from build123d import *

# Parameters (mm, degrees)
SKETCH_1_W          = 141
SKETCH_1_H          = 80
EXTRUDE_1_DEPTH     = 3
SKETCH_2_R          = 1.5
CUT_EXTRUDE_1_DEPTH = 4
SKETCH_3_R          = 1.5
CUT_EXTRUDE_2_DEPTH = 4


with BuildPart() as part:
    # ｽｹｯﾁ1 → ﾎﾞｽ - 押し出し1 (new body)
    with BuildSketch(Plane(origin=(0, 0, 0), x_dir=(1, 0, 0), z_dir=(0, 1, 0))):
        with Locations((-70.5, 40)):
            Rectangle(SKETCH_1_W, SKETCH_1_H)
    extrude(amount=EXTRUDE_1_DEPTH)

    # ｽｹｯﾁ2 → ｶｯﾄ - 押し出し1 (cut, through all)
    with BuildSketch(Plane(origin=(0, 3, 0), x_dir=(1, 0, 0), z_dir=(0, 1, 0))):
        with Locations(Location((-78.25, 75, 0), (0, 0, 270))):  # turned: the seam where the file's is
            Circle(SKETCH_2_R)
    extrude(amount=-CUT_EXTRUDE_1_DEPTH, mode=Mode.SUBTRACT)

    # ｽｹｯﾁ3 → ｶｯﾄ - 押し出し2 (cut, through all)
    with BuildSketch(Plane(origin=(0, 3, 0), x_dir=(1, 0, 0), z_dir=(0, 1, 0))):
        with Locations(Location((-62.75, 75, 0), (0, 0, 270))):  # turned: the seam where the file's is
            Circle(SKETCH_3_R)
    extrude(amount=-CUT_EXTRUDE_2_DEPTH, mode=Mode.SUBTRACT)


solid = part.part
Geometry check sheet. Reference: the model listing, model coordinates, mm. Round coordinates to 2 decimals unless told otherwise and drop trailing zeros. Write each loop counter-clockwise with the first axis right and the second up, starting at its lowest first coordinate (ties: lowest second). Pieces come first, ordered by that corner, then holes. Notation, with made-up numbers: (-36.5, 50) - (8.5, 50) arc R32 cw to (8.5, 86) - close; hole circle Ø4 at (87.25, 59). An arc over 180 degrees is marked (long way). One line per item, written item: value.
1. Cross-section at A-A on x = -62.75. Record the boundary of the cut face in (y, z).
The answers:
outline: (0, -80) - (3, -80) - (3, -76.5) - (0, -76.5) - close; (0, -73.5) - (3, -73.5) - (3, 0) - (0, 0) - close
2. Mould release check, pull along Z, two halves, no side actions. Record for faces 1 (the face through (-71, 1, -80)), 2 (the face through (-76.985, 1.521, -74.194)), 3 (the face through (-71, 1, 0)), 4 (the face through (-71, 3, -41)): released by +Z, released by -Z, zero draft, split by the parting line, or undercut.
The answers:
face 1: released by -Z
face 2: undercut
face 3: released by +Z
face 4: zero draft
3. Cross-section at B-B on z = -75. Record the boundary of the cut face in (x, y).
The answers:
outline: (-141, 0) - (-79.75, 0) - (-79.75, 3) - (-141, 3) - close; (-76.75, 0) - (-64.25, 0) - (-64.25, 3) - (-76.75, 3) - close; (-61.25, 0) - (0, 0) - (0, 3) - (-61.25, 3) - close
4. Depth check by flat-ended pin: pin 1 Ø4 at (x, z) = (-62.75, -75) entering from +Y. Enter the tip coordinate at first touch or a pass-through.
The answers:
pin 1: stops at y = 3
5. Scan lines: L1, parallel to X at y = 2.05, z = -75; L2, parallel to Z at x = -78.25, y = 1.35; L3, parallel to Z at x = -62, y = 0.8. Record each from-to range of solid material in increasing order.
The answers:
L1: x = -141 to -79.75, -76.75 to -64.25, -61.25 to 0
L2: z = -80 to -76.5, -73.5 to 0
L3: z = -80 to -76.3, -73.7 to 0
